Input: dimensioned drawing with shaded views. Units: mm. Origin: part minimum x, y, z. A direction names the side the tool comes from. Coordinates: 2 decimals unless noted, no trailing zeros. Loops run counter-clockwise (first coordinate to the right, second up) from the corner with the lowest first, then second, coordinate; pieces in that order, holes last.
Item 1: Section D-D on y = 101. Return loops of the section in (x, z).
Item 2: Section B-B on z = 24.5. Return loops of the section in (x, y) (1 decimal).
Item 3: Contact query for flat-ended pins moving along their axis: P1, Ø24, axis at y = 26, z = 33, coming from the +X side; P2, Ø12, axis at x = 51.5, z = 20, coming from the -Y side; P3, Ø5, axis at x = 34, z = 42, coming from the -Y side. Output: stop coordinate, or through.
Item 4: Ray query, line 1 along X through (y, z) = (12, 8.5); line 2 along X through (y, z) = (114, 94); line 3 along X through (y, z) = (61, 15). Return the intervals inside material, ascending.
Item 5: Section A-A on y = 31.5. Return loops of the section in (x, z).
Item 6: Pull-direction query (X, two-part tool) for the marked faces 3, 4, 5 and 6; classes: released by +X, released by -X, zero draft, split by the parting line, or undercut.
Item 7: Reachability of the marked faces 1 and 2 from +Z, -Z, +X, -X, +Y, -Y: full face, straight path, thin tool, end or side. Return the list, or none.
Item 8: Section C-C on x = 6. Return loops of the section in (y, z).
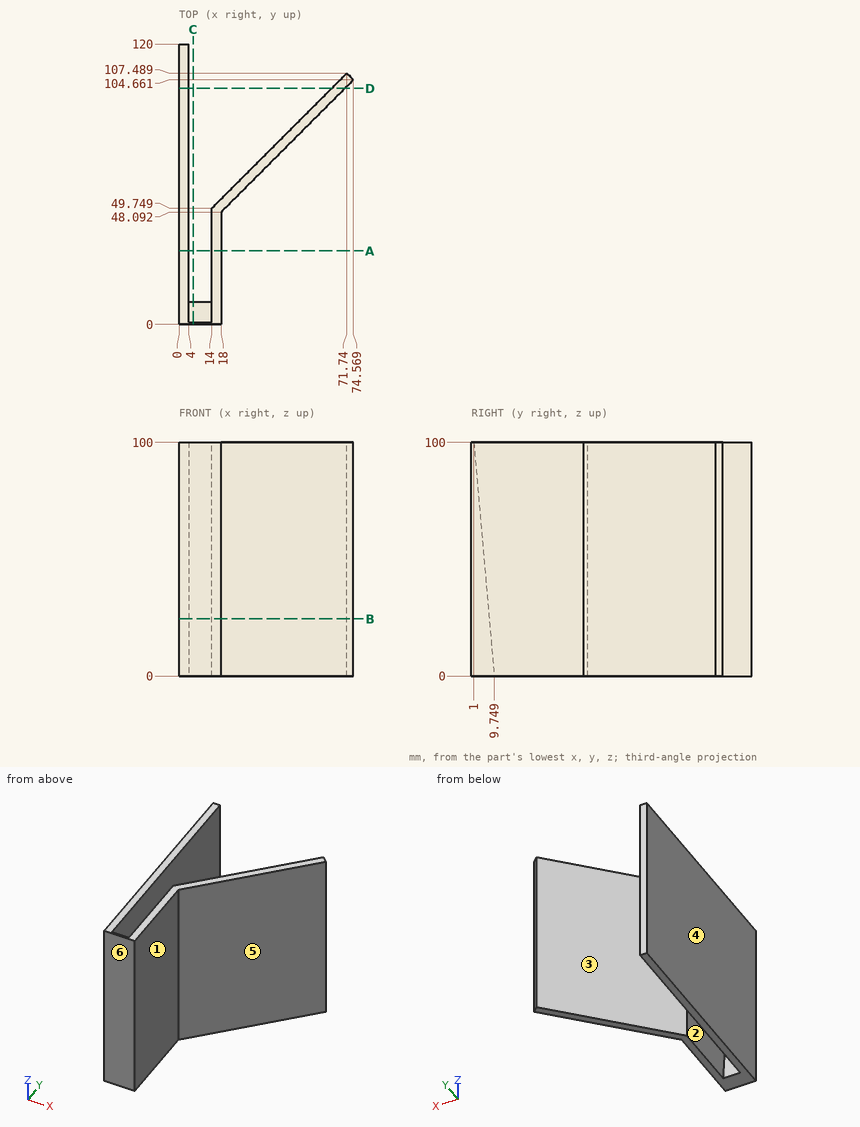
Results found:
1. outline: (0, 0) - (4, 0) - (4, 100) - (0, 100) - close; (65.25, 0) - (70.91, 0) - (70.91, 100) - (65.25, 100) - close
2. outline: (0, 0) - (18, 0) - (18, 48.1) - (74.6, 104.7) - (71.7, 107.5) - (14, 49.7) - (14, 7.6) - (4, 7.6) - (4, 120) - (0, 120) - close
3. P1: stops at x = 18
3. P2: stops at y = 75.59
3. P3: stops at y = 61.59
4. line 1: x = 0 to 4, 14 to 18
4. line 2: x = 0 to 4
4. line 3: x = 0 to 4, 25.25 to 30.91
5. outline: (0, 0) - (4, 0) - (4, 100) - (0, 100) - close; (14, 0) - (18, 0) - (18, 100) - (14, 100) - close
6. face 3: undercut
6. face 4: released by -X
6. face 5: released by +X
6. face 6: zero draft
7. face 1: +Z, -Z, +X, -Y
7. face 2: +Z, +Y
8. outline: (0, 0) - (9.75, 0) - (1, 100) - (0, 100) - close
